Work out the finished part from the listing and answer in its coordinate system (mm). A direction names the side the tool comes from. Round coordinates to 2 decimals unless told otherwise and drop trailing zeros. Loops run counter-clockwise (first coordinate to the right, second up) from the corner with the lowest first, then second, coordinate; pieces in that order, holes last.
from build123d import *

# Parameters (mm, degrees)
SKETCH_1_W          = 45.233636601
SKETCH_1_H          = 40
EXTRUDE_1_DEPTH     = 5
SKETCH_2_R          = 2.5
SKETCH_2_R_2        = 6.5
CUT_EXTRUDE_1_DEPTH = 6
SKETCH_3_W          = 45.2336366
SKETCH_3_H          = 40
EXTRUDE_2_DEPTH     = 5
EXTRUDE_3_DEPTH     = 45.233637
FILLET_1_R          = 3
FILLET_3_R          = 3
SKETCH_5_R          = 1.5
CUT_EXTRUDE_2_DEPTH = 6


with BuildPart() as part:
    # 草图1 → 凸台-拉伸1 (new body)
    with BuildSketch(Plane(origin=(-84.851927107, 0, -36.561705941), x_dir=(1, 0, 0), z_dir=(0, 1, 0))):
        with Locations((834.168962127, 191.534282172)):
            Rectangle(SKETCH_1_W, SKETCH_1_H)
    extrude(amount=EXTRUDE_1_DEPTH)

    # 草图2 → 切除-拉伸1 (cut, through all)
    with BuildSketch(Plane(origin=(0, 0, 0), x_dir=(-1, 0, 0), z_dir=(0, -1, 0))):
        with Locations((-766.81703502, 224.098378246)):
            Circle(SKETCH_2_R)
        with Locations((-731.81703502, 224.098378246)):
            Circle(SKETCH_2_R)
        with Locations((-749.31703502, 224.098378246)):
            Circle(SKETCH_2_R_2)
    extrude(amount=-CUT_EXTRUDE_1_DEPTH, mode=Mode.SUBTRACT)

    # 草图3 → 凸台-拉伸2 (add)
    with BuildSketch(Plane(origin=(0, 0, -248.095988113), x_dir=(-1, 0, 0), z_dir=(0, 0, -1))):
        with Locations((-749.31703502, 2.5)):
            Rectangle(SKETCH_3_W, SKETCH_3_H)
    extrude(amount=-EXTRUDE_2_DEPTH)

    # 草图4 → 凸台-拉伸3 (add)
    with BuildSketch(Plane.ZY.offset(-726.70021672)):
        Polygon((-232.73834126, 0), (-243.095988113, -8.75), (-243.095988113, 0), align=None)
    extrude(amount=-EXTRUDE_3_DEPTH)

    # 圆角1
    fillet_1_edges = [part.edges().sort_by_distance(p)[0] for p in [
        (771.93385332, 2.5, -208.095988113),
        (726.70021672, 2.5, -208.095988113),
    ]]
    fillet(fillet_1_edges, radius=FILLET_1_R)

    # 圆角3
    fillet_3_edges = [part.edges().sort_by_distance(p)[0] for p in [
        (726.70021672, 22.5, -245.595988113),
        (771.93385332, -17.5, -245.595988113),
        (771.93385332, 22.5, -245.595988113),
        (726.70021672, -17.5, -245.595988113),
    ]]
    fillet(fillet_3_edges, radius=FILLET_3_R)

    # 草图5 → 切除-拉伸2 (cut, through all)
    with BuildSketch(Plane.XY.offset(-243.095988113)):
        with Locations((763.31703502, 12.25)):
            Circle(SKETCH_5_R)
        with Locations((763.31703502, -11.625)):
            Circle(SKETCH_5_R)
        with Locations((735.31703502, -11.625)):
            Circle(SKETCH_5_R)
        with Locations((735.31703502, 12.25)):
            Circle(SKETCH_5_R)
    extrude(amount=-CUT_EXTRUDE_2_DEPTH, mode=Mode.SUBTRACT)


solid = part.part
Item 1: Straight lines are drawn through the part: line 1 (X direction, y = 12, z = -246); line 2 (Y direction, x = 738.5, z = -215); line 3 (Z direction, x = 739, y = 6.5). For each, find the intervals that lie inside material, in ascending order.
Item 2: For faces 5 (the face through (750, 14, -243.096)), 6 (the face through (750, -13, -243.096)), 7 (the face through (726.7, 1, -236)), determine the directions among +Z, -Z, +X, -X, +Y, -Y from which every point of the face is accessible in a straight line to the end or side of a thin tool.
Item 3: Section B-B, the plane z = -246 is taken. Give the vertices of the cut face in (x, y) (3 decimals).
Item 4: Section C-C, the plane x = 759.5 is taken. Give the vertices of the cut face in (y, z), plus the area to 3 significant figures.
Item 5: Section D-D, the plane z = -228 is taken. Give the vertices of the cut face in (x, y), plus the area to 3 significant figures.
Item 6: Section A-A, the plane y = 12.25 is taken. Give the vertices of the cut face in (x, z), plus the area to 3 significant figures.
Item 7: Each of these flat-tipped pins is pushed along its axis until it touches: P1, Ø5, axis at x = 763.32, y = 12.25, coming from the +Z side; P2, Ø6, axis at x = 737.5, y = -3.5, coming from the +Z side; P3, Ø8, axis at x = 766.82, z = -224.1, coming from the -Y side; P4, Ø4, axis at x = 740.5, z = -242, coming from the -Y side. Where does it stop, or does it pass through?
Item 8: Determine the mould class of faces 1 (the face through (771.078, 21.598, -245.561)), 2 (the face through (749, 0, -215)), 3 (the face through (736.75, 12.7, -245.56)), 4 (the face through (749, 2, -208.096)) for opening direction Y: pulls with the +Y half, pulls with the -Y half, needs draft (parallel to the pull), parting line crosses it, or undercut.
Answer below:
1. line 1: x = 726.7 to 733.84, 736.8 to 761.84, 764.8 to 771.93
1. line 2: y = 0 to 5
1. line 3: z = -248.1 to -243.1
2. face 5: +Z, +X, -X, +Y
2. face 6: +Z, +X, -X, -Y
2. face 7: +Z, -Z, -X, +Y, -Y
3. outline: (726.7, -14.5) arc R3 ccw to (729.7, -17.5) - (768.934, -17.5) arc R3 ccw to (771.934, -14.5) - (771.934, 19.5) arc R3 ccw to (768.934, 22.5) - (729.7, 22.5) arc R3 ccw to (726.7, 19.5) - close; hole circle Ø3 at (735.317, -11.625); hole circle Ø3 at (735.317, 12.25); hole circle Ø3 at (763.317, -11.625); hole circle Ø3 at (763.317, 12.25)
4. outline: (-17.5, -248.1) - (22.5, -248.1) - (22.5, -243.1) - (5, -243.1) - (5, -208.1) - (0, -208.1) - (0, -232.74) - (-8.75, -243.1) - (-17.5, -243.1) - close
4. area: 420 mm2
5. outline: (726.7, 0) - (744.12, 0) - (744.12, 5) - (726.7, 5) - close; (754.52, 0) - (771.93, 0) - (771.93, 5) - (754.52, 5) - close
5. area: 174 mm2
6. outline: (726.7, -248.1) - (733.82, -248.1) - (733.82, -243.1) - (726.7, -243.1) - close; (736.82, -248.1) - (761.82, -248.1) - (761.82, -243.1) - (736.82, -243.1) - close; (764.82, -248.1) - (771.93, -248.1) - (771.93, -243.1) - (764.82, -243.1) - close
6. area: 196 mm2
7. P1: stops at z = -243.1
7. P2: stops at z = -233.33
7. P3: stops at y = 0
7. P4: stops at y = -17.5
8. face 1: pulls with the +Y half
8. face 2: pulls with the -Y half
8. face 3: undercut
8. face 4: needs draft
